Geometry: see drawing. Coordinates: mm, zero at the bounding-box minimum. A direction names the side the tool comes from. Coordinates: 2 decimals unless noted, no trailing zeros. Write each loop counter-clockwise with the first axis right and the second up, starting at its lowest first coordinate (ties: lowest second). Pieces come first, ordered by that corner, then holes. Notation, with made-up numbers: M -27.75,-18.5 L -11.75,-18.5 A28 cw -11.75,-0.5 Z; hole C 15.5,6 d2. An arc over 180 degrees is marked long. Answer as CSV lines item,"result". Start each with the question number.
1. Section A-A on y = 114.3. Return the cut outline in (x, z), plus the area to 3 significant figures.
2. Reachability of the marked faces 4, 5 and 6 from +Z, -Z, +X, -X, +Y, -Y: full face, straight path, thin tool, end or side. Return the list, or none.
3. Line query: probe 1 along Y at (x, z) = (90, 114.3); probe 2 along Z at (x, y) = (56, 136.5); probe 3 along Y at (x, z) = (115.5, 93). Output: solid intervals per line, ascending. Write a range as [from, to].
4. Contact query for flat-ended pins moving along their axis: pin 1 Ø3 at (x, y) = (187.5, 148) entering from -Z; pin 2 Ø2 at (x, y) = (155, 105.5) entering from -Z; pin 3 Ø12 at (x, y) = (139, 196) entering from +Z. Output: stop coordinate, or through.
5. Section C-C on x = 121. Return the cut outline in (y, z).
6. Section D-D on z = 189. Return the cut outline in (x, y), plus the area to 3 significant figures.
7. Mould query, pull axis Y, two halves, no side actions, for the marked faces 1, 2 and 3. Classes: pulls with the +Y half, pulls with the -Y half, needs draft (parallel to the pull), parting line crosses it, or undercut.
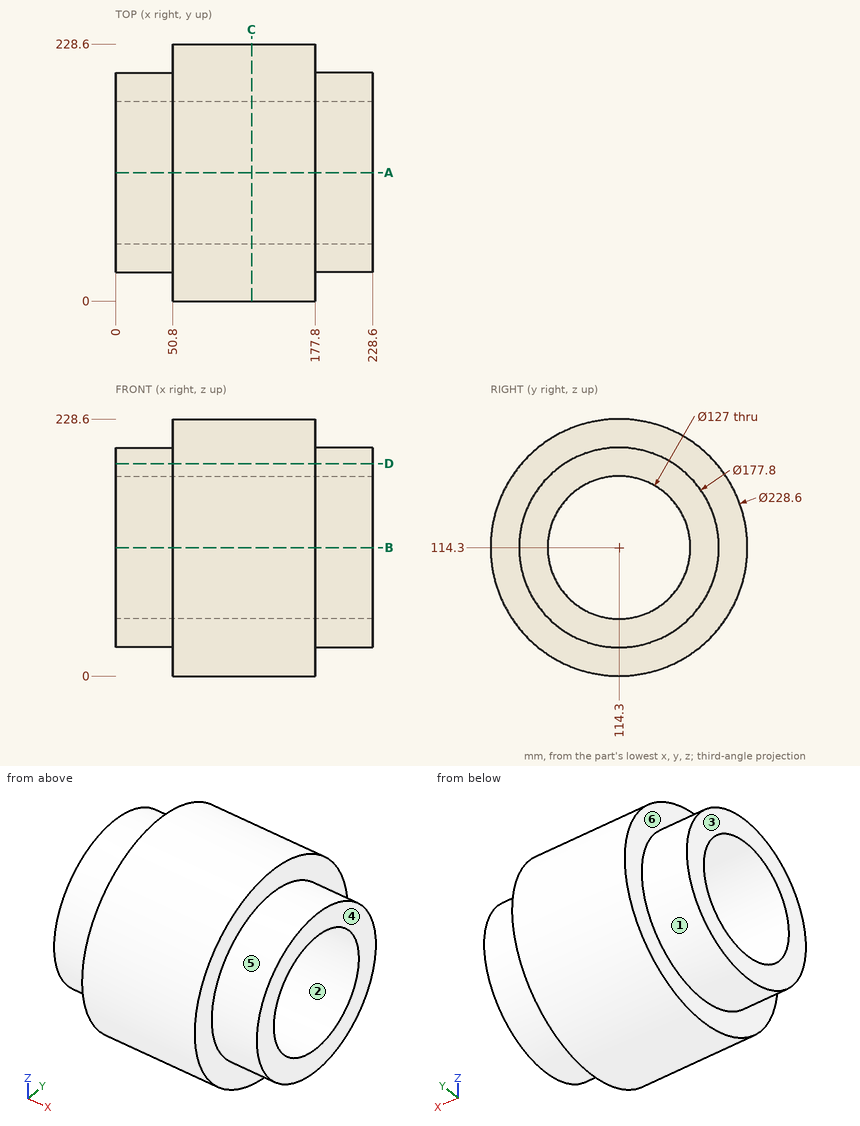
Values:
1,outline,"M 0,25.4 L 50.8,25.4 L 50.8,0 L 177.8,0 L 177.8,25.4 L 228.6,25.4 L 228.6,50.8 L 0,50.8 Z; M 0,177.8 L 228.6,177.8 L 228.6,203.2 L 177.8,203.2 L 177.8,228.6 L 50.8,228.6 L 50.8,203.2 L 0,203.2 Z"
1,area,"18,100 mm²"
2,face 4,"+Z, -Z, +X, +Y, -Y"
2,face 5,"+X"
2,face 6,"-X"
3,probe 1,"[0, 50.8], [177.8, 228.6]"
3,probe 2,"[2.18, 54.81], [173.79, 226.42]"
3,probe 3,"[2, 54.48], [174.12, 226.6]"
4,pin 1,"z = 31.44"
4,pin 2,"z = 0.27"
4,pin 3,"z = 199.94"
5,outline,"C 114.3,114.3 d228.6; hole C 114.3,114.3 d127"
6,outline,"M 0,66.1 L 50.8,66.1 L 50.8,27.79 L 177.8,27.79 L 177.8,66.1 L 228.6,66.1 L 228.6,162.5 L 177.8,162.5 L 177.8,200.81 L 50.8,200.81 L 50.8,162.5 L 0,162.5 Z"
6,area,"31,800 mm²"
7,face 1,"parting line crosses it"
7,face 2,"undercut"
7,face 3,"needs draft"
